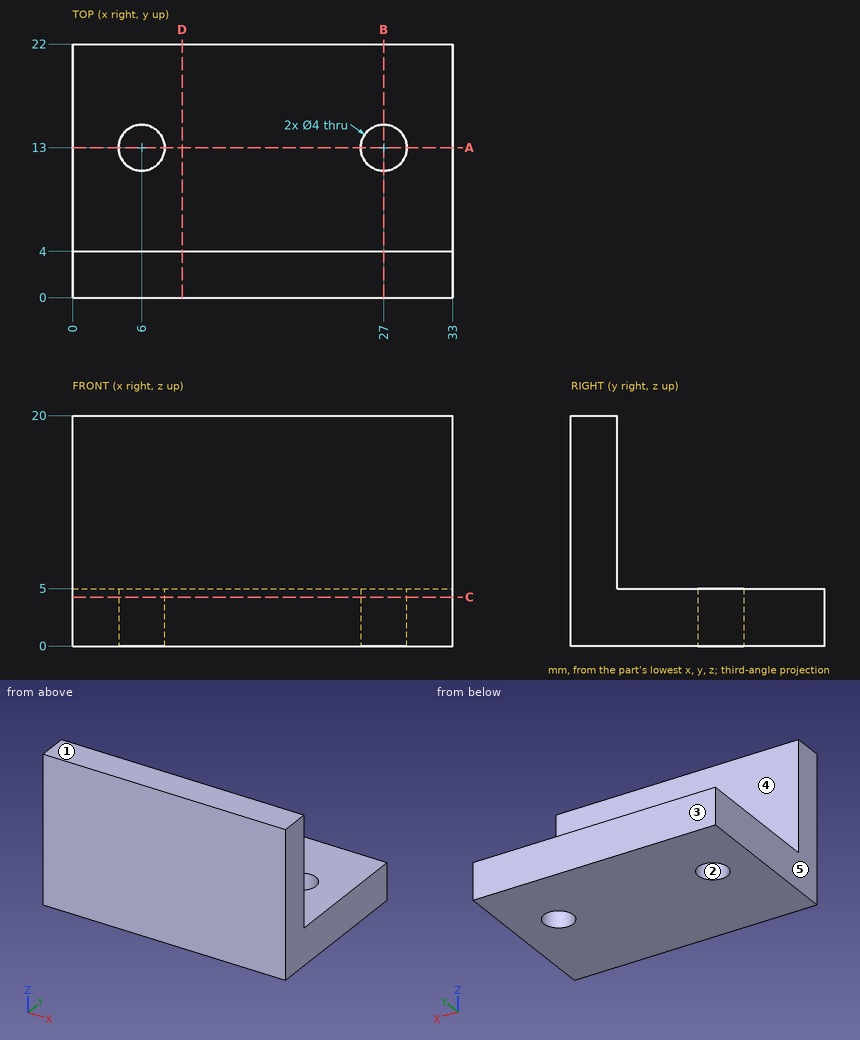
Check sheet for the drawn part. Datum: minimum x, y, z corner. Units: mm. A direction names the side the tool comes from. Coordinates: 2 decimals unless noted, no trailing zeros. Order: outer loops, then holes, each group sorted by start corner. A loop starts at its lowest first (then second) coordinate and runs counter-clockwise, first axis right, second up. Notation, with made-up numbers: M 65.5,68.25 L 93.5,68.25 A10 cw 93.5,80.25 Z; hole C 15.25,-25 d6. An arc over 180 degrees is marked long. One line per question, with ' | ' between items. Start each with the question number.
Item 1: Cross-section at C-C on z = 4.25. Enter the section's corners in (x, y), then the cut area to 3 significant figures.
Item 2: Draft check along Y on the marked faces 1, 2 and 3. Enter one of: pulls with the +Y half, pulls with the -Y half, needs draft (parallel to the pull), parting line crosses it, or undercut.
Item 3: Cross-section at A-A on y = 13. Enter the section's corners in (x, z), then the cut area to 3 significant figures.
Item 4: Gauge pin test, flat ends, axial feed: pin 1 (3 mm diameter, centred on x = 28.5, z = 7.5, fed in from +Y); pin 2 (5.5 mm diameter, centred on x = 20.5, y = 9, fed in from +Z). Record the tip position at first contact, or that the pin passes through.
Item 5: Cross-section at D-D on x = 9.5. Enter the section's corners in (y, z), then the cut area to 3 significant figures.
Item 6: Set-up check for the marked faces 4 and 5: record each of +Z, -Z, +X, -X, +Y, -Y from which the full face is reachable in a straight line by a thin tool's end or side.
Item 7: Material ranges on L1, parallel to X at y = 13, z = 2.7; L2, parallel to Y at x = 27, z = 2.5; L3, parallel to Y at x = 23, z = 15.5, recorded low to high. Write a range as [from, to].
Item 8: Cross-section at B-B on x = 27. Enter the section's corners in (y, z).
Findings:
1) outline: M 0,0 L 33,0 L 33,22 L 0,22 Z; hole C 6,13 d4; hole C 27,13 d4 | area: 701 mm²
2) face 1: needs draft | face 2: undercut | face 3: pulls with the +Y half
3) outline: M 0,0 L 4,0 L 4,5 L 0,5 Z; M 8,0 L 25,0 L 25,5 L 8,5 Z; M 29,0 L 33,0 L 33,5 L 29,5 Z | area: 125 mm²
4) pin 1: stops at y = 4 | pin 2: stops at z = 5
5) outline: M 0,0 L 22,0 L 22,5 L 4,5 L 4,20 L 0,20 Z | area: 170 mm²
6) face 4: +Z, +X, -X, +Y | face 5: +Z, -Z, -X, +Y, -Y
7) L1: x = [0, 4], [8, 25], [29, 33] | L2: y = [0, 11], [15, 22] | L3: y = [0, 4]
8) outline: M 0,0 L 11,0 L 11,5 L 4,5 L 4,20 L 0,20 Z; M 15,0 L 22,0 L 22,5 L 15,5 Z
